Verification items for the finished model (mm, model axes). Face numbers are marked on the shaded views. A direction names the side the tool comes from. Give positions to 0.01 mm unless a question says otherwise; leave off trailing zeros. Loops run counter-clockwise (first coordinate to the right, second up) from the corner with the lowest first, then second, coordinate; pieces in that order, holes last. Notation, with made-up numbers: (35.25, 81) -> (88.25, 81) arc R25 ccw to (88.25, 101) -> close; hole circle Ø6 at (26.5, 69). An arc over 180 degrees is marked (long way). Use one line per item in the form item = value. Start each with the question number.
from build123d import *

# Parameters (mm, degrees)
CUT_EXTRUDE1_DEPTH      = 24.3313898
CUT_EXTRUDE1_DEPTH_BACK = 24.3313898
SKETCH2_R               = 3.175


with BuildPart() as part:
    # Sketch1 → Revolve1 (revolve)
    with BuildSketch(Plane(origin=(0, 0, 0), x_dir=(0, 0, -1), z_dir=(1, 0, 0)), mode=Mode.PRIVATE) as revolve1_sk:
        Polygon((0, 0), (19.05, 0), (19.05, 3.175), (14.2875, 3.175), (14.2875, 9.525), (4.7625, 9.525), (4.7625, 3.175), (0, 3.175), align=None)
    revolve(revolve1_sk.sketch.rotate(Axis((0, 0, 0), (0, 0, -1)), 180), axis=Axis((0, 0, 0), (0, 0, -1)))

    # Sketch2 → Cut-Extrude1 (cut, two sides: drawn at the far end of the back side and taken through both)
    with BuildSketch(Plane(origin=(0, 0, 0), x_dir=(0, 0, -1), z_dir=(1, 0, 0)).offset(-CUT_EXTRUDE1_DEPTH_BACK)):
        with Locations((9.525, 0)):
            Circle(SKETCH2_R)
    extrude(amount=CUT_EXTRUDE1_DEPTH + CUT_EXTRUDE1_DEPTH_BACK, mode=Mode.SUBTRACT)


solid = part.part
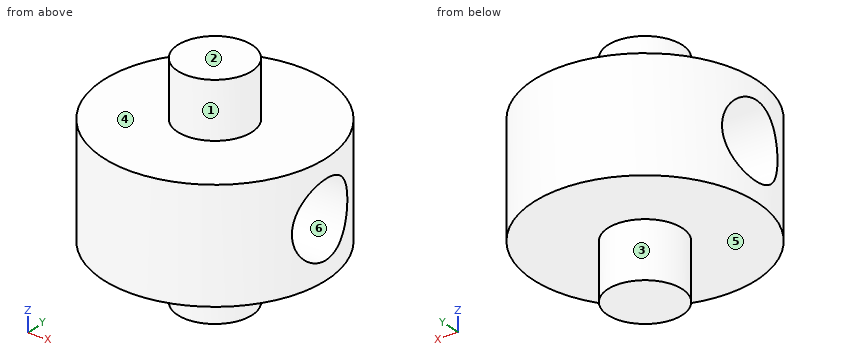
Item 1: Sectioned sample at D-D, the plane z = -2.5. Enter the section's corners in (x, y) (3 decimals).
Item 2: Gauge pin test, flat ends, axial feed: pin 1 Ø5 at (x, z) = (-3, -15.5) entering from -Y; pin 2 Ø6 at (x, y) = (-6, -3) entering from -Z; pin 3 Ø1 at (x, z) = (1, -5.5) entering from +Y. Record the tip position at first contact, or that the pin passes through.
Item 3: Tool access check on the marked faces 1, 2 and 3. Record the directions out of +Z, -Z, +X, -X, +Y, -Y that give a thin tool (end or side, any length) a straight path to the whole face; none if there is none.
Item 4: Draft check along Z on the marked faces 4, 5 and 6. Enter one of: +Z half, -Z half, draft (parallel to the pull), parting line (faces both ways), or undercut.
Item 5: Sectioned sample at C-C, the plane z = -6.75. Enter the section's corners in (x, y) (3 decimals), and give its area (3 significant figures).
Item 6: Material ranges on line 1 (Z direction, x = 4.5, y = 0); line 2 (Z direction, x = -0.5, y = 0); line 3 (Z direction, x = -5.5, y = -5.5), recorded low to high.
Outcome:
q1.outline = circle Ø6.35 at (0, 0)
q2.pin_1 = -9.49
q2.pin_2 = -14.29
q2.pin_3 = 9.51
q3.face_1 = +Z
q3.face_2 = +Z, +X, -X, +Y, -Y
q3.face_3 = -Z
q4.face_4 = +Z half
q4.face_5 = -Z half
q4.face_6 = undercut
q5.outline = (-9.399, -1.543) arc R9.525 ccw to (9.399, -1.543) -> close; (-9.399, 1.543) -> (9.399, 1.543) arc R9.525 ccw to start
q5.area = 227 mm^2
q6.line_1 = -14.29 to -12.7, -6.35 to -4.76
q6.line_2 = -19.05 to -12.7, -6.35 to 0
q6.line_3 = -14.29 to -4.76
